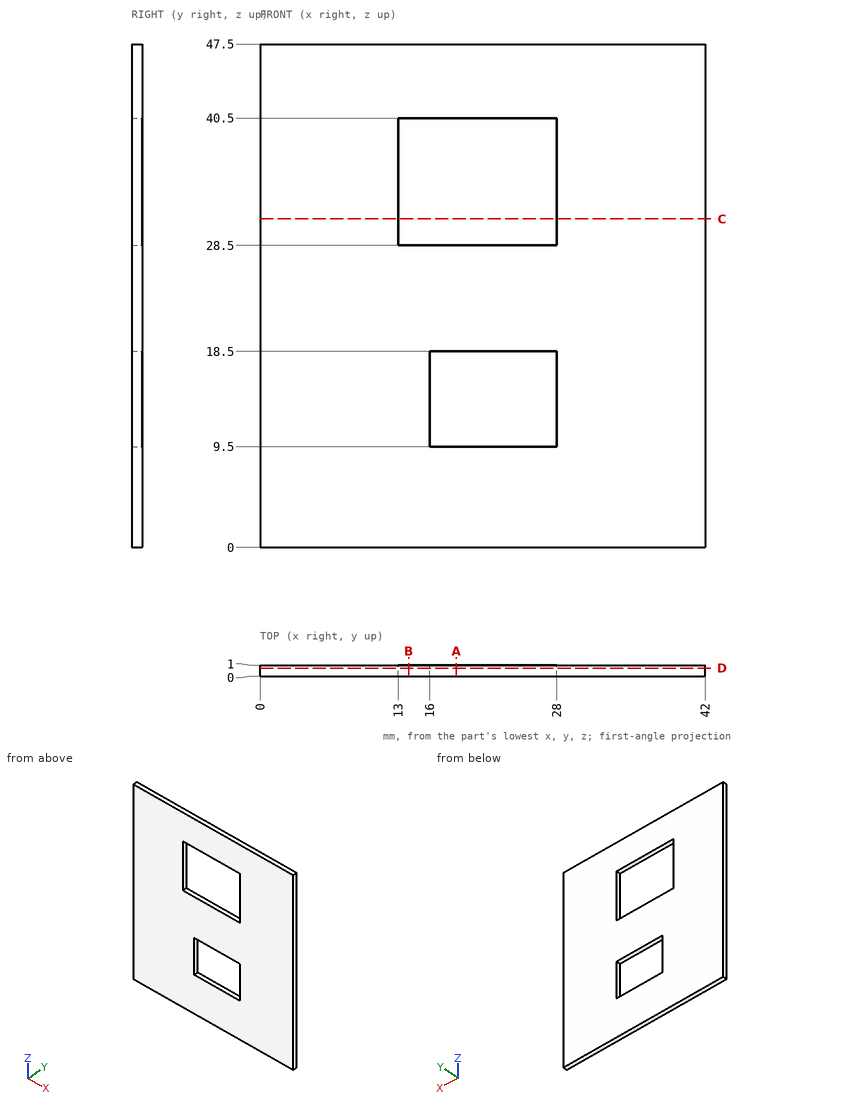
The figure shows three views and two pictorial views of one solid part (mm, origin at its lowest corner). Answer the questions. Round coordinates to 2 decimals unless told otherwise and drop trailing zeros. Loops run counter-clockwise (first coordinate to the right, second up) from the corner with the lowest first, then second, coordinate; pieces in that order, holes last. Notation, with made-up numbers: (6, -14.5) - (45, -14.5) arc R14 cw to (45, -7.5) - close; hole circle Ø3 at (69.5, 17). An arc over 180 degrees is marked (long way). Use one line per item in the form item = value. Start each with the question number.
(1) Find section A-A on x = 18.5. Determine the outline of the cut face in (y, z).
(2) Find section B-B on x = 14. Determine the outline of the cut face in (y, z).
(3) Consider line 1 (X direction, y = 0.5, z = 12.5); line 2 (X direction, y = 0.6, z = 30.5); line 3 (Z direction, x = 15, y = 0.8). Determine where each line is inside the solid, lowest interval first.
(4) Find section C-C on z = 31. Determine the outline of the cut face in (x, y), and give its area (3 significant figures).
(5) Find section D-D on y = 0.75. Determine the outline of the cut face in (x, z).
Answer list:
q1.outline = (0, 0) - (1, 0) - (1, 9.5) - (0, 9.5) - close; (0, 18.5) - (1, 18.5) - (1, 28.5) - (0, 28.5) - close; (0, 40.5) - (1, 40.5) - (1, 47.5) - (0, 47.5) - close
q2.outline = (0, 0) - (1, 0) - (1, 28.5) - (0, 28.5) - close; (0, 40.5) - (1, 40.5) - (1, 47.5) - (0, 47.5) - close
q3.line_1 = 0 to 16, 28 to 42
q3.line_2 = 0 to 13, 28 to 42
q3.line_3 = 0 to 28.5, 40.5 to 47.5
q4.outline = (0, 0) - (13, 0) - (13, 1) - (0, 1) - close; (28, 0) - (42, 0) - (42, 1) - (28, 1) - close
q4.area = 27.0 mm^2
q5.outline = (0, 0) - (42, 0) - (42, 47.5) - (0, 47.5) - close; hole (13, 28.5) - (28, 28.5) - (28, 40.5) - (13, 40.5) - close; hole (16, 9.5) - (28, 9.5) - (28, 18.5) - (16, 18.5) - close
